from build123d import *

# Parameters (mm, degrees)
SKETCH1_W           = 7
SKETCH1_H           = 7
SKETCH1_R           = 2
BOSS_EXTRUDE1_DEPTH = 1.6
SKETCH5_OUTSIDE_W   = 25.63
SKETCH5_OUTSIDE_H   = 25.63
SKETCH5_OUTSIDE_R   = 3.5
CUT_EXTRUDE2_DEPTH  = 4.2
CUT_EXTRUDE2_TAPER  = 60


with BuildPart() as part:
    # Sketch1 → Boss-Extrude1 (new body, symmetric)
    with BuildSketch(Plane(origin=(0, 0, 0), x_dir=(1, 0, 0), z_dir=(0, 1, 0))):
        Rectangle(SKETCH1_W, SKETCH1_H)
        Circle(SKETCH1_R, mode=Mode.SUBTRACT)
    extrude(amount=BOSS_EXTRUDE1_DEPTH, both=True)

    # Sketch5 outside → Cut-Extrude2 (cut, through all)
    with BuildSketch(Plane(origin=(0, 1.6, 0), x_dir=(1, 0, 0), z_dir=(0, 1, 0))):
        Rectangle(SKETCH5_OUTSIDE_W, SKETCH5_OUTSIDE_H)
        Circle(SKETCH5_OUTSIDE_R, mode=Mode.SUBTRACT)
    extrude(amount=-CUT_EXTRUDE2_DEPTH, taper=CUT_EXTRUDE2_TAPER, mode=Mode.SUBTRACT)


solid = part.part
Design review of the part built by this model. Coordinates are the model's own, in mm. Round coordinates to 2 decimals unless told otherwise and drop trailing zeros. Write each loop counter-clockwise with the first axis right and the second up, starting at its lowest first coordinate (ties: lowest second). Pieces come first, ordered by that corner, then holes. Notation, with made-up numbers: (62, 37.5) - (120, 37.5) arc R21 cw to (120, 55.5) - close; hole circle Ø8 at (87, -10). An arc over 180 degrees is marked (long way). Return JSON: item names as keys, results as strings. Group by question number.
Item 1: For probe 1 along Z at (x, y) = (0, -0.4); probe 2 along Z at (x, y) = (1.75, 0.5), list the stretches that pass through material, from the lowest coordinate up. Write a range as [from, to].
Item 2: We need section B-B on y = 1.4. Write out the cut boundary in (x, z).
Item 3: We need section C-C on y = 1. Write out the cut boundary in (x, z).
Item 4: We need section A-A on y = 0. Write out the cut boundary in (x, z).
Item 5: The part is to be moulded in two halves that separate along Z. For faces 1 (the face through (-2, -1.6, 2)), 2 (the face through (0, 0, 2)), 3 (the face through (0, 0, 3.5)), say which applies: pulls with the +Z half, pulls with the -Z half, needs draft (parallel to the pull), parting line crosses it, or undercut.
Model answer:
{
 "1": {"probe 1": "z = [-3.5, -2], [2, 3.5]", "probe 2": "z = [-3.5, -0.97], [0.97, 3.5]"},
 "2": {"outline": "(-3.5, -1.6) arc R3.85 ccw to (-1.6, -3.5) - (1.6, -3.5) arc R3.85 ccw to (3.5, -1.6) - (3.5, 1.6) arc R3.85 ccw to (1.6, 3.5) - (-1.6, 3.5) arc R3.85 ccw to (-3.5, 1.6) - close; hole circle Ø4 at (0, 0)"},
 "3": {"outline": "(-3.5, -2.89) arc R4.54 ccw to (-2.89, -3.5) - (2.89, -3.5) arc R4.54 ccw to (3.5, -2.89) - (3.5, 2.89) arc R4.54 ccw to (2.89, 3.5) - (-2.89, 3.5) arc R4.54 ccw to (-3.5, 2.89) - close; hole circle Ø4 at (0, 0)"},
 "4": {"outline": "(-3.5, -3.5) - (3.5, -3.5) - (3.5, 3.5) - (-3.5, 3.5) - close; hole circle Ø4 at (0, 0)"},
 "5": {"face 1": "needs draft", "face 2": "undercut", "face 3": "pulls with the +Z half"}
}
